Verification items for this drawing (mm, ordinates from the low corner). Round coordinates to 2 decimals unless told otherwise and drop trailing zeros. Order: outer loops, then holes, each group sorted by start corner. A loop starts at its lowest first (then second) coordinate and runs counter-clockwise, first axis right, second up.
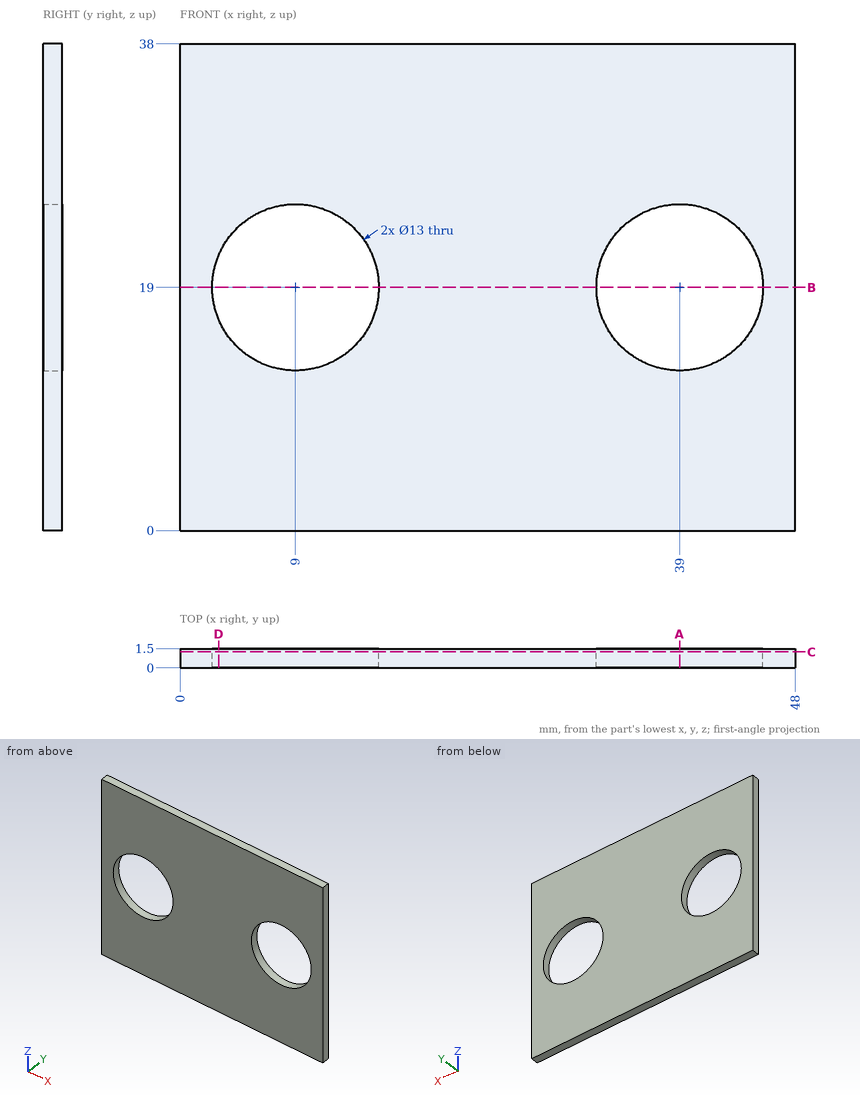
Item 1: Scan lines: line 1 along Z through (x, y) = (9, 0.8); line 2 along X through (y, z) = (0.35, 24); line 3 along Z through (x, y) = (7, 1.4). Record each from-to range of solid material in increasing order.
Answer:
line 1: z = 0 to 12.5, 25.5 to 38
line 2: x = 0 to 4.85, 13.15 to 34.85, 43.15 to 48
line 3: z = 0 to 12.82, 25.18 to 38
Item 2: Sectioned sample at C-C (y = 1.25). Record the cut outline in (x, z), and give its area (3 significant figures).
Answer:
outline: (0, 0) - (48, 0) - (48, 38) - (0, 38) - close; hole circle Ø13 at (9, 19); hole circle Ø13 at (39, 19)
area: 1,560 mm2
Item 3: Sectioned sample at D-D (x = 3). Record the cut outline in (y, z).
Answer:
outline: (0, 0) - (1.5, 0) - (1.5, 16.5) - (0, 16.5) - close; (0, 21.5) - (1.5, 21.5) - (1.5, 38) - (0, 38) - close
Item 4: Sectioned sample at A-A (x = 39). Record the cut outline in (y, z).
Answer:
outline: (0, 0) - (1.5, 0) - (1.5, 12.5) - (0, 12.5) - close; (0, 25.5) - (1.5, 25.5) - (1.5, 38) - (0, 38) - close
Item 5: Sectioned sample at B-B (z = 19). Record the cut outline in (x, y).
Answer:
outline: (0, 0) - (2.5, 0) - (2.5, 1.5) - (0, 1.5) - close; (15.5, 0) - (32.5, 0) - (32.5, 1.5) - (15.5, 1.5) - close; (45.5, 0) - (48, 0) - (48, 1.5) - (45.5, 1.5) - close
